For this review, take the finished solid that the model builds, in its own axes (mm). A direction names the side the tool comes from. Coordinates: 2 decimals unless noted, no trailing zeros. Loops run counter-clockwise (first coordinate to the right, second up) from the corner with the lowest first, then second, coordinate; pieces in that order, holes last. Notation, with made-up numbers: (3, -29.5) - (17, -29.5) arc R26 cw to (17, 7.5) - close; hole circle Ø6 at (34.5, 79). An arc over 180 degrees is marked (long way). Answer as a JSON object with one key per item and string values. Group by question number.
Item 1: We need section A-A (y = 4.5). Give the boundary of the cut face in (x, z).
Item 2: To check wall thickness, follow line 1 (Y direction, x = 6, z = 1.5); line 2 (Y direction, x = 9.1, z = 3); line 3 (Z direction, x = 26, y = 35.5). State the ranges of each line that lie inside material, in increasing order.
Item 3: Tool access review of faces 1 (the flat face through (27.575, 1, 3)), 2 (the flat face through (27, -0.5, 3)), 3 (the flat face through (9, 2, 4)), 4 (the flat face through (27, 21, -1)), 5 (the flat face through (2, 21, 4)): name each direction out of +Z, -Z, +X, -X, +Y, -Y from which nothing blocks a thin tool from reaching the whole face with its end or side.
Item 4: We need section C-C (y = 19). Give the boundary of the cut face in (x, z).
Item 5: Clearance check with flat-ended pins moving along their axes: pin 1 (1.5 mm diameter, centred on y = 19, z = 3.5, fed in from -X); pin 2 (1.5 mm diameter, centred on x = 23.5, z = 5, fed in from +Y); pin 3 (1.5 mm diameter, centred on x = 9.5, z = 4, fed in from -Y). State where each tip first meets the part, or that it passes through.
Item 6: We need section D-D (x = 35). Give the boundary of the cut face in (y, z), then the cut area to 3 significant figures.
Item 7: We need section B-B (x = 8.1). Give the boundary of the cut face in (y, z), then the cut area to 3 significant figures.
Item 8: Mouldability with a two-part tool opening along Y and no side actions: class faces 6 (the flat face through (15.2, 21, 4)), 7 (the flat face through (20, -0.5, 3)), 8 (the cylindrical face through (11.869, 3.277, 2.549)) as released by +Y, released by -Y, zero draft, split by the parting line, or undercut.
from build123d import *

# Parameters (mm, degrees)
SKETCH_1_W           = 17.2
SKETCH_1_H           = 42
SKETCH_1_W_2         = 13.2
SKETCH_1_H_2         = 38
EXTRUDE_1_DEPTH      = 1
SKETCH_2_W           = 1
SKETCH_2_H           = 10
EXTRUDE_2_DEPTH      = 2.5
EXTRUDE_3_DEPTH      = 2.5
EXTRUDE_3_DEPTH_BACK = 2.5
EXTRUDE_4_DEPTH      = 2.5
EXTRUDE_4_DEPTH_BACK = 2.5
SKETCH_5_W           = 60.014732212
SKETCH_5_H           = 45
EXTRUDE_5_DEPTH      = 1
FILLET_1_R           = 2
SKETCH_6_W           = 8.55
SKETCH_6_H           = 3.5
EXTRUDE_6_DEPTH      = 6.3
SKETCH_7_W           = 3.972075094
SKETCH_7_H           = 1
EXTRUDE_7_DEPTH      = 6.3
SKETCH_8_R           = 6
CUT_EXTRUDE_1_DEPTH  = 72.978746863
EXTRUDE_START        = 6
SKETCH_9_W           = 13.2
SKETCH_9_H           = 38
SKETCH_9_R           = 6
EXTRUDE_8_DEPTH      = 6
FILLET_2_R           = 0.15
SKETCH_10_W          = 6.3
SKETCH_10_H          = 3.5
CUT_EXTRUDE_2_DEPTH  = 0.2


with BuildPart() as part:
    # 草图1 → 凸台-拉伸1 (new body)
    with BuildSketch(Plane.XY):
        with Locations((8.6, 21)):
            Rectangle(SKETCH_1_W, SKETCH_1_H)
        with Locations((8.6, 21)):
            Rectangle(SKETCH_1_W_2, SKETCH_1_H_2, mode=Mode.SUBTRACT)
    extrude(amount=EXTRUDE_1_DEPTH)

    # 草图2 → 凸台-拉伸2 (add)
    with BuildSketch(Plane.XY.offset(1)):
        with Locations((16.7, 34)):
            Rectangle(SKETCH_2_W, SKETCH_2_H)
        with Locations((0.5, 8)):
            Rectangle(SKETCH_2_W, SKETCH_2_H)
    extrude(amount=EXTRUDE_2_DEPTH)

    # 草图3 → 凸台-拉伸3 (add, two sides: drawn at the far end of the back side and taken through both)
    with BuildSketch(Plane(origin=(0, 34, 0), x_dir=(-1, 0, 0), z_dir=(0, -1, 0)).offset(-EXTRUDE_3_DEPTH_BACK)):
        with BuildLine():
            Line((-17.2, -1.75), (-17.2, -2.75))
            ThreePointArc((-17.2, -2.75), (-17.7, -2.25), (-17.2, -1.75))
        make_face()
    extrude(amount=EXTRUDE_3_DEPTH + EXTRUDE_3_DEPTH_BACK)

    # 草图4 → 凸台-拉伸4 (add, two sides: drawn at the far end of the back side and taken through both)
    with BuildSketch(Plane(origin=(0, 8, 0), x_dir=(-1, 0, 0), z_dir=(0, -1, 0)).offset(-EXTRUDE_4_DEPTH_BACK)):
        with BuildLine():
            Line((0, -1.75), (0, -2.75))
            ThreePointArc((0, -2.75), (0.129409523, -2.732962913), (0.25, -2.683012702))
            Line((0.25, -2.683012702), (0.25, -1.816987298))
            ThreePointArc((0.25, -1.816987298), (0.129409523, -1.767037087), (0, -1.75))
        make_face()
    extrude(amount=EXTRUDE_4_DEPTH + EXTRUDE_4_DEPTH_BACK)

    # 草图5 → 凸台-拉伸5 (add)
    with BuildSketch(Plane(origin=(0, 0, 0), x_dir=(-1, 0, 0), z_dir=(0, 0, -1))):
        with Locations((-26.992633894, 21)):
            Rectangle(SKETCH_5_W, SKETCH_5_H)
    extrude(amount=EXTRUDE_5_DEPTH)

    # 圆角1
    fillet_1_edges = [part.edges().sort_by_distance(p)[0] for p in [
        (57, 43.5, -0.5),
        (57, -1.5, -0.5),
        (-3.014732212, -1.5, -0.5),
        (-3.014732212, 43.5, -0.5),
    ]]
    fillet(fillet_1_edges, radius=FILLET_1_R)

    # 草图6 → 凸台-拉伸6 (add)
    with BuildSketch(Plane.XY):
        with Locations((23.5, 1.25)):
            Rectangle(SKETCH_6_W, SKETCH_6_H)
    extrude(amount=EXTRUDE_6_DEPTH)

    # 草图7 → 凸台-拉伸7 (add)
    with BuildSketch(Plane.XY):
        with Locations((23.516201891, -1)):
            Rectangle(SKETCH_7_W, SKETCH_7_H)
    extrude(amount=EXTRUDE_7_DEPTH)

    # 草图8 → 切除-拉伸1 (cut, through all)
    with BuildSketch(Plane.XY):
        with Locations((9.1, 8.6)):
            Circle(SKETCH_8_R)
        with Locations((8.1, 33.4)):
            Circle(SKETCH_8_R)
    extrude(amount=-CUT_EXTRUDE_1_DEPTH, mode=Mode.SUBTRACT)

    # 草图9 → 凸台-拉伸8 (add)
    with BuildSketch(Plane.XY.offset(EXTRUDE_START)):
        with Locations((8.6, 21)):
            Rectangle(SKETCH_9_W, SKETCH_9_H)
        with Locations((9.1, 8.6)):
            Circle(SKETCH_9_R, mode=Mode.SUBTRACT)
        with Locations((8.1, 33.4)):
            Circle(SKETCH_9_R, mode=Mode.SUBTRACT)
    extrude(amount=-EXTRUDE_8_DEPTH)

    # 圆角2
    fillet_2_edges = [part.edges().sort_by_distance(p)[0] for p in [
        (-0.25, 8, 1.816987298),
        (-0.25, 8, 2.683012702),
    ]]
    fillet(fillet_2_edges, radius=FILLET_2_R)

    # 草图10 → 切除-拉伸2 (cut)
    with BuildSketch(Plane(origin=(27.775, 0, 0), x_dir=(0, 0, -1), z_dir=(1, 0, 0))):
        with Locations((-3.15, 1.25)):
            Rectangle(SKETCH_10_W, SKETCH_10_H)
    extrude(amount=-CUT_EXTRUDE_2_DEPTH, mode=Mode.SUBTRACT)


solid = part.part
Check sheet entries:
{
 "1": {"outline": "(-3.01, -1) - (4.72, -1) - (4.72, 6) - (2, 6) - (2, 1) - (1, 1) - (1, 3.5) - (0, 3.5) - (0, 0) - (-3.01, 0) - close; (13.48, -1) - (57, -1) - (57, 0) - (17.2, 0) - (17.2, 1) - (15.2, 1) - (15.2, 6) - (13.48, 6) - close"},
 "2": {"line 1": "y = 2 to 3.46, 13.74 to 27.78, 39.02 to 40", "line 2": "y = 2 to 2.6, 14.6 to 27.48, 39.32 to 40", "line 3": "z = -1 to 0"},
 "3": {"face 1": "+Z, +X, +Y, -Y", "face 2": "+Z, +X, -Y", "face 3": "+Z, -X, -Y", "face 4": "-Z, +X, -X, +Y, -Y", "face 5": "+Z, +Y, -Y"},
 "4": {"outline": "(-3.01, -1) - (57, -1) - (57, 0) - (17.2, 0) - (17.2, 1) - (15.2, 1) - (15.2, 6) - (2, 6) - (2, 1) - (0, 1) - (0, 0) - (-3.01, 0) - close"},
 "5": {"pin 1": "stops at x = 2", "pin 2": "stops at y = 3", "pin 3": "stops at y = 2"},
 "6": {"outline": "(-1.5, -1) - (43.5, -1) - (43.5, 0) - (-1.5, 0) - close", "area": "45.0 mm2"},
 "7": {"outline": "(-1.5, -1) - (2.68, -1) - (2.68, 6) - (2, 6) - (2, 1) - (0, 1) - (0, 0) - (-1.5, 0) - close; (14.52, -1) - (27.4, -1) - (27.4, 6) - (14.52, 6) - close; (39.4, -1) - (43.5, -1) - (43.5, 0) - (42, 0) - (42, 1) - (40, 1) - (40, 6) - (39.4, 6) - close", "area": "110 mm2"},
 "8": {"face 6": "zero draft", "face 7": "released by -Y", "face 8": "undercut"}
}
